Read the model definition and answer for the solid it produces. Units are mm, in the model's axes. A direction names the side the tool comes from. Give positions to 0.01 mm unless a question says otherwise; leave off trailing zeros. Write each loop counter-clockwise with the first axis right and the second up, starting at its lowest first coordinate (ties: lowest second). Pieces come first, ordered by that corner, then holes.
```python
from build123d import *

# Parameters (mm, degrees)
SKETCH1_R           = 11.45
BOSS_EXTRUDE1_DEPTH = 57.5
SKETCH2_R           = 7.45
BOSS_EXTRUDE2_DEPTH = 15
CUT_EXTRUDE1_DEPTH  = 15


with BuildPart() as part:
    # Sketch1 → Boss-Extrude1 (new body)
    with BuildSketch(Plane(origin=(0, 0, 0), x_dir=(1, 0, 0), z_dir=(0, 1, 0))):
        with Locations(Location((0, 0, 0), (0, 0, 270))):
            Circle(SKETCH1_R)
    extrude(amount=BOSS_EXTRUDE1_DEPTH)

    # Sketch2 → Boss-Extrude2 (add)
    with BuildSketch(Plane(origin=(0, 57.5, 0), x_dir=(1, 0, 0), z_dir=(0, 1, 0))):
        with Locations(Location((0, 0, 0), (0, 0, 270))):
            Circle(SKETCH2_R)
    extrude(amount=BOSS_EXTRUDE2_DEPTH)

    # Sketch3 → Cut-Extrude1 (cut)
    with BuildSketch(Plane.XZ):
        with BuildLine():
            Line((1.547024754, 3.742888511), (-3.474906974, 2.080269579))
            ThreePointArc((-3.474906974, 2.080269579), (-1.079149377, -3.903579975), (4.05, 0))
            ThreePointArc((4.05, 0), (3.366596965, 2.251338462), (1.547024754, 3.742888511))
        make_face()
    extrude(amount=-CUT_EXTRUDE1_DEPTH, mode=Mode.SUBTRACT)


solid = part.part
```
Item 1: Section D-D (y = 24.5) is taken. Write down the section's boundary in (x, z).
Result set:
outline: circle Ø22.9 at (0, 0)
Item 2: Section C-C (z = -5.5) is taken. Write down the section's boundary in (x, y).
Result set:
outline: (-10.04, 0) - (10.04, 0) - (10.04, 57.5) - (5.03, 57.5) - (5.03, 72.5) - (-5.03, 72.5) - (-5.03, 57.5) - (-10.04, 57.5) - close
Item 3: Section A-A (y = 12) is taken. Write down the section's boundary in (x, z).
Result set:
outline: circle Ø22.9 at (0, 0); hole (-3.47, 2.08) arc R4.05 ccw (long way) to (1.55, 3.74) - close
Item 4: Which of the six approach directions +Z, -Z, +X, -X, +Y, -Y give full straight-line access (tool end or side, diameter ignored) to faces 4 (the flat face through (0, 72.5, 0)), 5 (the flat face through (-0.929, 7.395, 2.923)), 6 (the flat face through (-2.4, 57.5, 7.5))?
Result set:
face 4: +Z, -Z, +X, -X, +Y
face 5: -Y
face 6: +Y
Item 5: Find the intervals of material crossed by line 1 along X through (y, z) = (8, 0); line 2 along Y through (x, z) = (7.5, -5.5); line 3 along Z through (x, y) = (-3.5, 4.5), in increasing order.
Result set:
line 1: x = -11.45 to -4.05, 4.05 to 11.45
line 2: y = 0 to 57.5
line 3: z = -10.9 to -2.04, 2.04 to 10.9
Item 6: Determine the mould class of faces 1 (the flat face through (-5, 0, 0)), 2 (the flat face through (0, 15, 0)), 3 (the cylindrical face through (-11.18, 28.35, -2.48)) for opening direction X: pulls with the +X half, pulls with the -X half, needs draft (parallel to the pull), parting line crosses it, or undercut.
Result set:
face 1: needs draft
face 2: undercut
face 3: parting line crosses it
Item 7: Each of these flat-tipped pins is pushed along its axis until it touches: pin 1 Ø4 at (y, z) = (31, 8) entering from -X; pin 2 Ø3 at (x, y) = (4.5, 18) entering from -Z; pin 3 Ø3 at (x, z) = (-9, 1) entering from +Y. Where does it stop, or does it pass through?
Result set:
pin 1: stops at x = -9.75
pin 2: stops at z = -11.05
pin 3: stops at y = 57.5
Item 8: Section B-B (x = 0) is taken. Write down the section's boundary in (y, z), and give its area (3 significant figures).
Result set:
outline: (0, -11.45) - (57.5, -11.45) - (57.5, -7.45) - (72.5, -7.45) - (72.5, 7.45) - (57.5, 7.45) - (57.5, 11.45) - (0, 11.45) - (0, 3.23) - (15, 3.23) - (15, -4.05) - (0, -4.05) - close
area: 1,430 mm2
